Can you work these out from the drawing? Everything is in mm from the part's minimum corner. A direction names the side the tool comes from. Give positions to 0.01 mm unless a question says otherwise; leave off trailing zeros. Order: outer loops, then holes, each group sorted by start corner. A loop starts at its lowest first (then second) coordinate and runs counter-clockwise, first axis right, second up. Notation, with made-up numbers: (64, 48) -> (105, 48) arc R23 cw to (105, 64) -> close; hole circle Ø5 at (89.5, -36). An arc over 180 degrees is marked (long way). Answer as CSV lines item,"result". Start each with the question number.
(1) I want a section at B-B (x = 9). Please give me the cut outline in (y, z) (1 decimal).
(2) On a 3-axis mill with a long thin cutter (end or side, diameter ignored), from which of +Z, -Z, +X, -X, +Y, -Y can I reach the whole of each face in a straight line? I mean the marked faces 5, 6 and 7. Say none if no direction works.
(3) I need wall thicknesses on L1, parallel to Z at x = 9.25, y = 19; L2, parallel to X at y = 16, z = 18; L3, parallel to Z at x = 1.5, y = 25. Which ranges of each line are inside material? Lowest first, please.
(4) I want a section at C-C (z = 17.5). Please give me the cut outline in (x, y).
(5) I want a section at A-A (y = 18.5). Please give me the cut outline in (x, z).
(6) We'd pull the mould along Y, two halves only. Please class the marked faces 1, 2, 3 and 4: released by +Y, released by -Y, zero draft, split by the parting line, or undercut.
(7) Will these pins go through, and if not, where does the flat tip stop? pin 1 Ø5 at (y, z) = (21, 9) entering from -X; pin 2 Ø5.5 at (y, z) = (15, 18) entering from +X; pin 3 Ø1 at (x, y) = (5, 26) entering from +Z.
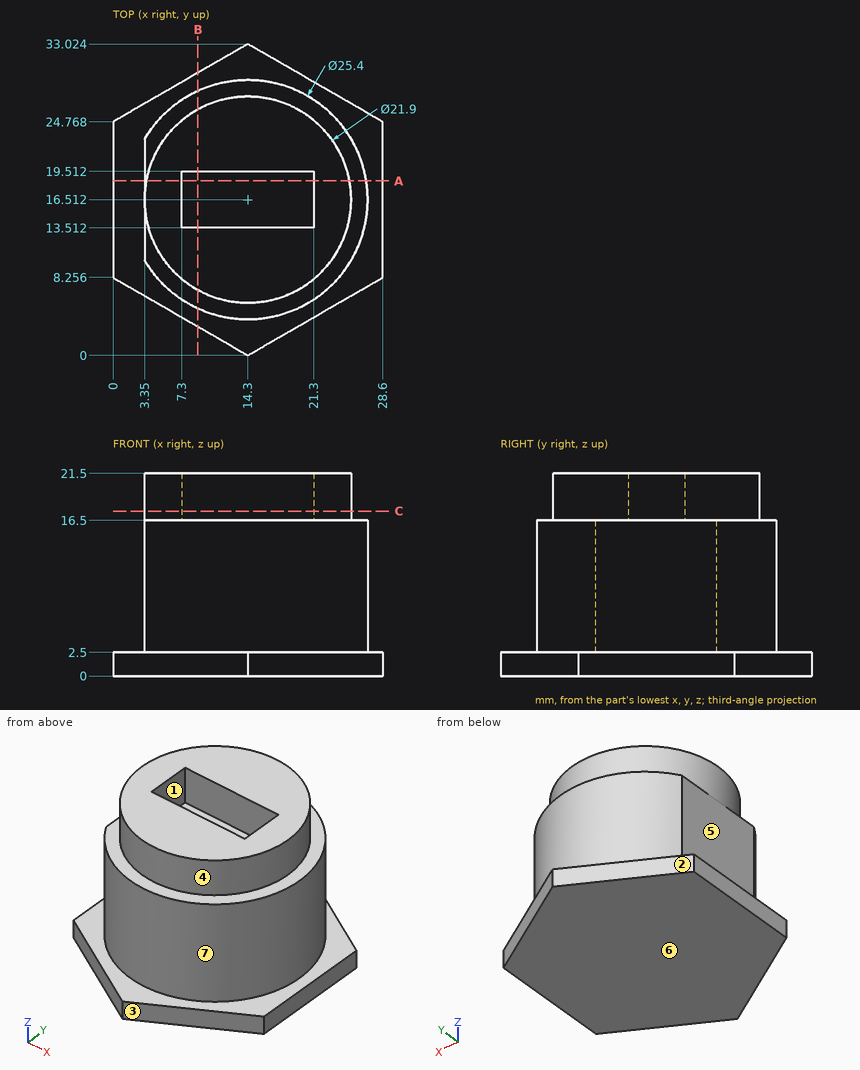
Final values:
1,outline,"(3.1, 0) -> (30, 0) -> (30, 2.5) -> (28.1, 2.5) -> (28.1, 16.5) -> (26.1, 16.5) -> (26.1, 21.5) -> (19.5, 21.5) -> (19.5, 16.5) -> (13.5, 16.5) -> (13.5, 21.5) -> (6.9, 21.5) -> (6.9, 16.5) -> (5, 16.5) -> (5, 2.5) -> (3.1, 2.5) -> close"
2,face 5,"+Z, -X, +Y, -Y"
2,face 6,"-Z, +X, -X, +Y, -Y"
2,face 7,"+Z"
3,L1,"0 to 16.5"
3,L2,"3.36 to 7.3, 21.3 to 25.24"
3,L3,"0 to 2.5"
4,outline,"circle Ø21.9 at (14.3, 16.51); hole (7.3, 13.51) -> (21.3, 13.51) -> (21.3, 19.51) -> (7.3, 19.51) -> close"
5,outline,"(0, 0) -> (28.6, 0) -> (28.6, 2.5) -> (26.84, 2.5) -> (26.84, 16.5) -> (25.07, 16.5) -> (25.07, 21.5) -> (21.3, 21.5) -> (21.3, 16.5) -> (7.3, 16.5) -> (7.3, 21.5) -> (3.53, 21.5) -> (3.53, 16.5) -> (3.35, 16.5) -> (3.35, 2.5) -> (0, 2.5) -> close"
6,face 1,"undercut"
6,face 2,"released by +Y"
6,face 3,"released by -Y"
6,face 4,"split by the parting line"
7,pin 1,"x = 3.35"
7,pin 2,"x = 27"
7,pin 3,"z = 2.5"
